```python
from build123d import *

# Parameters (mm, degrees)
F2_R     = 3.25
F3_DEPTH = 3
F4_R     = 1.75
F5_DEPTH = 32.894


with BuildPart() as f1:
    # F0 (on Right) → F1 (revolve)
    with BuildSketch(Plane.YZ):
        Polygon((1.6256, 17.399), (0, 17.399), (0, 11.0744), (1.5748, 11.0744), (1.5748, 12.5984), (3.0734, 12.5984), (3.0734, 11.0744), (10.21715, 11.0744), (10.21715, 8.7884), (26.546713, 8.7884), (28.1305, 7.874), (32.893, 7.874), (32.893, 15.875), (10.0076, 15.875), (10.0076, 25.146), (5.2324, 25.146), (5.2324, 17.399), (3.7592, 17.399), (3.7592, 15.875), (1.6256, 15.875), align=None)
    revolve(axis=Axis((0, 16.4465, 0), (0, 1, 0)))

    # F2 (on face) → F3 (cut)
    with BuildSketch(Plane(origin=(0, 10.0076, 0), x_dir=(-1, 0, 0), z_dir=(0, 1, 0))):
        with Locations((0, 20.7264)):
            Circle(F2_R)
        with Locations((-14.655778, 14.655778)):
            Circle(F2_R)
        with Locations((-20.7264, 0)):
            Circle(F2_R)
        with Locations((-14.655778, -14.655778)):
            Circle(F2_R)
        with Locations((0, -20.7264)):
            Circle(F2_R)
        with Locations((14.655778, -14.655778)):
            Circle(F2_R)
        with Locations((20.7264, 0)):
            Circle(F2_R)
        with Locations((14.655778, 14.655778)):
            Circle(F2_R)
    extrude(amount=-F3_DEPTH, mode=Mode.SUBTRACT)

    # F4 (on Front) → F5 (cut, through all)
    with BuildSketch(Plane.XZ):
        with Locations((0, 20.7264)):
            Circle(F4_R)
        with Locations((-14.655778, 14.655778)):
            Circle(F4_R)
        with Locations((-20.7264, 0)):
            Circle(F4_R)
        with Locations((-14.655778, -14.655778)):
            Circle(F4_R)
        with Locations((0, -20.7264)):
            Circle(F4_R)
        with Locations((14.655778, -14.655778)):
            Circle(F4_R)
        with Locations((20.7264, 0)):
            Circle(F4_R)
        with Locations((14.655778, 14.655778)):
            Circle(F4_R)
    extrude(amount=-F5_DEPTH, mode=Mode.SUBTRACT)


solid = f1.part
```
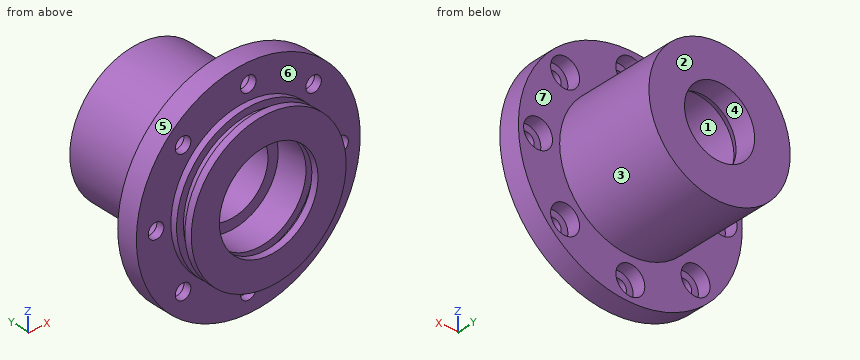
The model under review builds one solid part; all positions refer to its coordinate system, in mm. Face numbers are marked on the shaded views. A direction names the side the tool comes from. Round coordinates to 2 decimals unless told otherwise and drop trailing zeros. Order: outer loops, then holes, each group sorted by start corner. A loop starts at its lowest first (then second) coordinate and runs counter-clockwise, first axis right, second up.
Item 1: To check wall thickness, follow probe 1 along Y at (x, z) = (-13, -12); probe 2 along Y at (x, z) = (-2.5, -11.5); probe 3 along Z at (x, y) = (2, 29). State the ranges of each line that lie inside material, in increasing order.
Working result:
probe 1: y = 5.23 to 7.01
probe 2: y = 0 to 1.57, 3.07 to 32.89
probe 3: z = -15.75 to -7.62, 7.62 to 15.75
Item 2: Add section A-A, the plane x = 20.5. State the section outline as (y, z) points.
Working result:
outline: (5.23, -14.56) - (10.01, -14.56) - (10.01, -3.24) - (7.01, -3.24) - (7.01, -1.74) - (5.23, -1.74) - close; (5.23, 1.74) - (7.01, 1.74) - (7.01, 3.24) - (10.01, 3.24) - (10.01, 14.56) - (5.23, 14.56) - close
Item 3: Machinability: for the marked faces 5, 6 and 7, which of the approach directions +Z, -Z, +X, -X, +Y, -Y give a long, thin tool a straight path to every point of the face, cutting with its end or side? Answer none if there is none.
Working result:
face 5: +Y, -Y
face 6: -Y
face 7: +Y
Item 4: For pin 1 (12 mm diameter, centred on y = 25, z = 1.5, fed in from -X) (3 decimals); pin 2 (3 mm diameter, centred on x = 16, z = -15.5, fed in from +Y); pin 3 (8.5 mm diameter, centred on x = -14.66, z = 14.66, fed in from +Y), all flat-tipped, find the tip position at first contact; note any pin that passes through.
Working result:
pin 1: stops at x = -15.875
pin 2: stops at y = 7.01
pin 3: stops at y = 10.01
Item 5: Draft analysis for pull direction X (two halves, no side actions). For the marked faces 1, 2, 3 and 4, state which applies: released by +X, released by -X, zero draft, split by the parting line, or undercut.
Working result:
face 1: undercut
face 2: zero draft
face 3: split by the parting line
face 4: undercut
Item 6: Add section C-C, the plane x = 0. Count the separate pieces of the cut face and the enclosed holes in it, and give its area (3 significant figures).
Working result:
separate pieces: 4
enclosed holes: 0
area: 472 mm2
Item 7: Add section B-B, the plane y = 12. State the section outline as (x, z) points (3 decimals).
Working result:
outline: circle Ø31.75 at (0, 0); hole circle Ø17.577 at (0, 0)
